For this review, take the finished solid that the model builds, in its own axes (mm). A direction names the side the tool comes from. Coordinates: 2 decimals unless noted, no trailing zeros. Loops run counter-clockwise (first coordinate to the right, second up) from the corner with the lowest first, then second, coordinate; pieces in that order, holes last.
Autodesk Inventor part; units mm, degrees
ref_plane "YZ Plane" through (0, 0, 0) normal (1, 0, 0) x (0, 1, 0)
ref_plane "XZ Plane" through (0, 0, 0) normal (0, 1, 0) x (-1, 0, 0)
ref_plane "XY Plane" through (0, 0, 0) normal (0, 0, 1) x (1, 0, 0)
sketch "Sketch1" plane through (0, 0, 0) normal (0, 1, 0) x (-1, 0, 0)
  line L0 (17.7, -17.15) -> (-17.7, -17.15)
  line L1 (-17.7, -17.15) -> (-17.7, 17.15)
  line L2 (-17.7, 17.15) -> (17.7, 17.15)
  line L3 (17.7, 17.15) -> (17.7, -17.15)
  line L4 (28.56, 0) -> (-28.56, 0)
  line L5 (0, -27.79) -> (0, 27.79)
  line L6 (-3.7, 7.15) -> (6.3, 7.15)
  line L7 (6.3, 7.15) -> (6.3, -7.15)
  line L8 (6.3, -7.15) -> (-3.7, -7.15)
  line L9 (-3.7, -15.15) -> (-3.7, -7.15)
  line L10 (-3.7, 7.15) -> (-3.7, 15.15)
  line L11 (15.7, 15.15) -> (-3.7, 15.15)
  line L12 (-3.7, -15.15) -> (15.7, -15.15)
  line L13 (15.7, -15.15) -> (15.7, 15.15)
  line L14 (-18.4, -17.85) -> (18.4, -17.85)
  line L15 (18.4, -17.85) -> (18.4, 17.85)
  line L16 (18.4, 17.85) -> (-18.4, 17.85)
  line L17 (-18.4, 17.85) -> (-18.4, -17.85)
  line L18 (20.4, -19.85) -> (-20.4, -19.85)
  line L19 (-20.4, -19.85) -> (-20.4, 19.85)
  line L20 (-20.4, 19.85) -> (20.4, 19.85)
  line L21 (20.4, 19.85) -> (20.4, -19.85)
  point P0 (0, 0)
  dimension "d0" = 34.3
  dimension "d1" = 35.4
  dimension "d3" = 10
  dimension "d4" = 10
  dimension "d5" = 24
  dimension "d6" = 14
  dimension "d7" = 14
  dimension "d8" = 2
  dimension "d9" = 2
  dimension "d10" = 2
  dimension "d11" = 0.7
  dimension "d12" = 2
extrude "Extrusion1" add sketch "Sketch1" along normal blind 4 contours L3 L4 L15 L14 L5 L0 | L0 L5 L12 L13 L4 L3 | L5 L14 L17 L4 L1 L0 | L0 L1 L4 L5 L8 L9 L12 | L4 L13 L11 L5 L2 L3 | L3 L2 L5 L16 L15 L4 | L14 L15 L4 L21 L18 L5 | L5 L18 L19 L4 L17 L14 | L15 L16 L5 L20 L21 L4 | L4 L17 L16 L5 L2 L1 | L1 L2 L5 L11 L10 L6 L4 | L5 L4 L7 L8 | L4 L5 L6 L7 | L4 L19 L20 L5 L16 L17
extrude "Extrusion2" add sketch "Sketch1" against normal blind 2 contours L14 L15 L4 L21 L18 L5 | L5 L18 L19 L4 L17 L14 | L15 L16 L5 L20 L21 L4 | L4 L19 L20 L5 L16 L17
sketch "Sketch3" plane through (0, 4, 0) normal (0, 1, 0) x (1, 0, 0)
  line L0 (-28.56, 0) -> (28.56, 0)
  line L1 (0, 27.79) -> (0, -27.79)
  circle A0 centre (0, 0) radius 4
  dimension "d17" = 8
extrude "Extrusion3" cut sketch "Sketch3" against normal blind 4
properties part number "cam_socket"
Q1. Machinability: for faces 1 (the face through (0, 1, 19.85)), 2 (the face through (18.4, -1, 0)), 3 (the face through (-6, 2, 15.15)), which of the approach directions +Z, -Z, +X, -X, +Y, -Y give a long, thin tool a straight path to every point of the face, cutting with its end or side? Answer none if there is none.
Q2. Consider section D-D (z = 14). State the section outline as (x, y) points, then the cut area to 3 significant figures.
Q3. Consider section C-C (x = 0). State the section outline as (y, z) points, then the cut area to 3 significant figures.
Q4. The part is to be moulded in two halves that separate along X. For faces 4 (the face through (3.7, 2, -11)), 5 (the face through (5, 4, 0)), 6 (the face through (-20.4, 1, 0)), 7 (the face through (20.4, 1, 0)), say which applies: +X half, -X half, draft (parallel to the pull), parting line (faces both ways), or undercut.
Q5. For pin 1 Ø8 at (x, z) = (10, 12.5) entering from -Y; pin 2 Ø5 at (x, z) = (0, 0) entering from +Y, all flat-tipped, find the tip position at first contact; note any pin that passes through.
Q6. Consider section B-B (y = 2.75). State the section outline as (x, z) points, then the cut area to 3 significant figures.
Q7. Consider section A-A (z = 0). State the section outline as (x, y) points, then the cut area to 3 significant figures.
Q8. Wall thickness on probe 1 along Z at (x, y) = (0, 2.75); probe 2 along X at (y, z) = (1.4, 0); probe 3 along Z at (x, y) = (-4.5, 2.4): over which ranges is each line inside the solid? List them lowest first.
Model answer:
1. face 1: +Z, +X, -X, +Y, -Y
1. face 2: -Y
1. face 3: +Y, -Y
2. outline: (-20.4, -2) - (-18.4, -2) - (-18.4, 0) - (-15.7, 0) - (-15.7, 4) - (-20.4, 4) - close; (3.7, 0) - (18.4, 0) - (18.4, -2) - (20.4, -2) - (20.4, 4) - (3.7, 4) - close
2. area: 93.6 mm2
3. outline: (-2, -19.85) - (4, -19.85) - (4, -15.15) - (0, -15.15) - (0, -17.85) - (-2, -17.85) - close; (-2, 17.85) - (0, 17.85) - (0, 15.15) - (4, 15.15) - (4, 19.85) - (-2, 19.85) - close; (0, -7.15) - (4, -7.15) - (4, -4) - (0, -4) - close; (0, 4) - (4, 4) - (4, 7.15) - (0, 7.15) - close
3. area: 70.8 mm2
4. face 4: undercut
4. face 5: draft
4. face 6: -X half
4. face 7: +X half
5. pin 1: stops at y = 0
5. pin 2: passes through
6. outline: (-20.4, -19.85) - (20.4, -19.85) - (20.4, 19.85) - (-20.4, 19.85) - close; hole (-15.7, -15.15) - (3.7, -15.15) - (3.7, -7.15) - (-6.3, -7.15) - (-6.3, 7.15) - (3.7, 7.15) - (3.7, 15.15) - (-15.7, 15.15) - close; hole circle Ø8 at (0, 0)
6. area: 1,120 mm2
7. outline: (-20.4, -2) - (-18.4, -2) - (-18.4, 0) - (-15.7, 0) - (-15.7, 4) - (-20.4, 4) - close; (-6.3, 0) - (-4, 0) - (-4, 4) - (-6.3, 4) - close; (4, 0) - (18.4, 0) - (18.4, -2) - (20.4, -2) - (20.4, 4) - (4, 4) - close
7. area: 102 mm2
8. probe 1: z = -19.85 to -15.15, -7.15 to -4, 4 to 7.15, 15.15 to 19.85
8. probe 2: x = -20.4 to -15.7, -6.3 to -4, 4 to 20.4
8. probe 3: z = -19.85 to -15.15, -7.15 to 7.15, 15.15 to 19.85
